Model file for the job. Use its own axes, mm. A direction names the side the tool comes from. Round coordinates to 2 decimals unless told otherwise and drop trailing zeros. Loops run counter-clockwise (first coordinate to the right, second up) from the corner with the lowest first, then second, coordinate; pieces in that order, holes last. Notation, with made-up numbers: (80.5, -21.75) - (116.5, -21.75) arc R25 cw to (116.5, 1.25) - close; hole circle Ø2 at (79.5, 73). An arc over 180 degrees is marked (long way). Answer as a JSON object with one key per item and string values.
from build123d import *

# Parameters (mm, degrees)
F0_W     = 101.6
F0_H     = 21.59
F1_DEPTH = 6.35
F2_W     = 22.733
F2_H     = 12.319
F3_DEPTH = 25.4
F4_W     = 22.86
F4_H     = 1.7018
F5_DEPTH = 7.112
F6_W     = 22.86
F6_H     = 1.7018
F7_DEPTH = 7.112
F9_D     = 3.81


with BuildPart() as f1:
    # F0 (on Front) → F1 (new body)
    with BuildSketch(Plane.XZ):
        with Locations((4.648548, 21.848283)):
            Rectangle(F0_W, F0_H)
    extrude(amount=F1_DEPTH)

    # F2 (on face) → F3 (cut)
    with BuildSketch(Plane.XZ.offset(6.35)):
        with Locations((-23.608952, 22.064183)):
            Rectangle(F2_W, F2_H)
        with Locations((32.906048, 22.064183)):
            Rectangle(F2_W, F2_H)
    extrude(amount=-F3_DEPTH, mode=Mode.SUBTRACT)

    # F4 (on face) → F5 (join)
    with BuildSketch(Plane.XZ.offset(6.35)):
        with Locations((4.648548, 11.904183)):
            Rectangle(F4_W, F4_H)
    extrude(amount=F5_DEPTH)

    # F6 (on Front) → F7 (join)
    with BuildSketch(Plane.XZ):
        with Locations((4.648548, 11.904183)):
            Rectangle(F6_W, F6_H)
    extrude(amount=-F7_DEPTH)

    # F9 (through all)
    with Locations(Plane.XY.offset(12.755083)):
        with Locations((-2.971452, 3.556), (12.268548, 3.556), (12.268548, -9.906), (-2.971452, -9.906)):
            Hole(F9_D / 2)


solid = f1.part
1) Slice it at A-A on x = 32. List the corners of the cut face in (y, z), then the cut area to 3 significant figures.
Values follow:
{"outline": "(-6.35, 11.05) - (0, 11.05) - (0, 15.9) - (-6.35, 15.9) - close; (-6.35, 28.22) - (0, 28.22) - (0, 32.64) - (-6.35, 32.64) - close", "area": "58.9 mm²"}
2) Probe probe 1 along X at (y, z) = (-4, 27.5); probe 2 along Z at (x, y) = (-27, -4.25); probe 3 along Y at (x, z) = (13, 12). List the from-to ranges inside material, lowest first.
Values follow:
{"probe 1": "-46.15 to -34.98, -12.24 to 21.54, 44.27 to 55.45", "probe 2": "11.05 to 15.9, 28.22 to 32.64", "probe 3": "-13.46 to -11.66, -8.15 to 1.8, 5.31 to 7.11"}
3) Tool access for faces 4 (the flat face through (-6.781, -10, 12)), 5 (the flat face through (-24, -3, 28.224)), 6 (the flat face through (4, 4, 12.755)), 7 (the flat face through (-6.781, 4, 12)): list every direction of +Z, -Z, +X, -X, +Y, -Y with a clear straight run to the whole face (end or side of a thin tool).
Values follow:
{"face 4": "+Z, -Z, -X, -Y", "face 5": "+Y, -Y", "face 6": "+Z, +X, -X, +Y", "face 7": "+Z, -Z, -X, +Y"}
4) Slice it at C-C on x = 0. List the corners of the cut face in (y, z), then the cut area to 3 significant figures.
Values follow:
{"outline": "(-13.46, 11.05) - (7.11, 11.05) - (7.11, 12.76) - (0, 12.76) - (0, 32.64) - (-6.35, 32.64) - (-6.35, 12.76) - (-13.46, 12.76) - close", "area": "161 mm²"}
5) Two-plate mould, pull along Z, no slides. Class faces 1 (the flat face through (4, -10, 12.755)), 2 (the flat face through (33, -3, 28.224)), 3 (the flat face through (16.079, 4, 12)): pulls with the +Z half, pulls with the -Z half, needs draft (parallel to the pull), parting line crosses it, or undercut.
Values follow:
{"face 1": "pulls with the +Z half", "face 2": "undercut", "face 3": "needs draft"}
6) Drop flat-ended pins along their axis: P1, Ø0.9, axis at y = 3, z = 11.5, coming from the +X side; P2, Ø11, axis at x = 19, z = 24.5, coming from the -Y side; P3, Ø1, axis at x = -0.5, z = 23.5, coming from the +Y side. Give the stop position or say it passes through.
Values follow:
{"P1": "x = 16.08", "P2": "y = -6.35", "P3": "y = 0"}
7) Slice it at B-B on z = 23.75. List the corners of the cut face in (x, y).
Values follow:
{"outline": "(-46.15, -6.35) - (-34.98, -6.35) - (-34.98, 0) - (-46.15, 0) - close; (-12.24, -6.35) - (21.54, -6.35) - (21.54, 0) - (-12.24, 0) - close; (44.27, -6.35) - (55.45, -6.35) - (55.45, 0) - (44.27, 0) - close"}
8) Slice it at D-D on y = -3.25. List the corners of the cut face in (x, z).
Values follow:
{"outline": "(-46.15, 11.05) - (55.45, 11.05) - (55.45, 32.64) - (-46.15, 32.64) - close; hole (-34.98, 15.9) - (-12.24, 15.9) - (-12.24, 28.22) - (-34.98, 28.22) - close; hole (21.54, 15.9) - (44.27, 15.9) - (44.27, 28.22) - (21.54, 28.22) - close"}
